Source: CAD feature listing. Evaluate the final solid. Frame: model axes, mm. Face numbers are marked on the shaded views. Coordinates: 2 decimals unless noted, no trailing zeros. Loops run counter-clockwise (first coordinate to the right, second up) from the corner with the lowest first, then second, coordinate; pieces in that order, holes last. Notation, with made-up numbers: (42, 43) - (59, 43) arc R18 ccw to (59, 59) - close; hole circle Ø5 at (60.5, -15). An arc over 180 degrees is marked (long way). Write item = value, one per line. Start each with the question number.
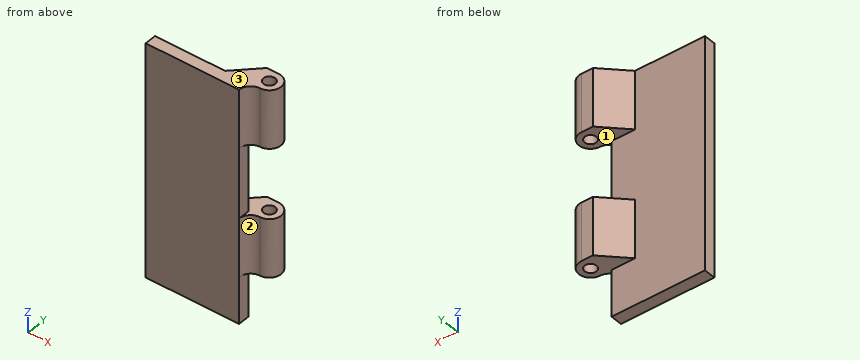
from build123d import *

# Parameters (mm, degrees)
SKETCH1_W              = 8
SKETCH1_H              = 20
BOSS_EXTRUDE1_DEPTH    = 1
SKETCH2_R              = 0.5
BOSS_EXTRUDE2_DEPTH    = 5
FILLET1_R              = 1
LPATTERN1_COUNT        = 2
LPATTERN1_PITCH        = 11
FILLET1_OF_LPATTERN1_R = 1


with BuildPart() as part:
    # Sketch1 → Boss-Extrude1 (new body)
    with BuildSketch(Plane(origin=(0, 0, 0), x_dir=(1, 0, 0), z_dir=(0, 1, 0))):
        with Locations((4, 10)):
            Rectangle(SKETCH1_W, SKETCH1_H)
    extrude(amount=BOSS_EXTRUDE1_DEPTH)

    # Sketch2 → Boss-Extrude2 (add)
    with BuildSketch(Plane.XY):
        with BuildLine():
            Line((8, 1), (9, 1))
            ThreePointArc((9, 1), (10, 2), (9, 3))
            Line((9, 3), (8, 3))
            Line((8, 3), (6, 1))
            Line((6, 1), (8, 1))
        make_face()
        with Locations((9, 2)):
            Circle(SKETCH2_R, mode=Mode.SUBTRACT)
    boss_extrude2 = extrude(amount=-BOSS_EXTRUDE2_DEPTH)

    # Fillet1
    fillet1_edges = [part.edges().sort_by_distance(p)[0] for p in [
        (8, 1, -2.5),
    ]]
    fillet(fillet1_edges, radius=FILLET1_R - 0.0001)  # a hair under: the kernel refuses the full size

    # LPattern1: Boss-Extrude2 ×2
    with Locations(*[(0, 0, -i * LPATTERN1_PITCH) for i in range(1, LPATTERN1_COUNT)]):
        add(boss_extrude2)

    # Fillet1 of LPattern1
    fillet1_of_lpattern1_edges = [part.edges().sort_by_distance(p)[0] for p in [
        (8, 1, -13.5),
    ]]
    fillet(fillet1_of_lpattern1_edges, radius=FILLET1_OF_LPATTERN1_R - 0.0001)  # a hair under: the kernel refuses the full size


solid = part.part
Item 1: Cut plane B-B (x = 5). Return the cut outline in (y, z).
Item 2: Material intervals for L1, parallel to Y at x = 9, z = -1.55; L2, parallel to Z at x = 7.5, y = 2.45; L3, parallel to Y at x = 1.75, z = -4.75, sorted ascending. Write a range as [from, to].
Item 3: Cut plane A-A (y = 2). Return the cut outline in (x, z), then the cut area to 3 significant figures.
Item 4: Draft query along Z for the marked faces 1, 2 and 3. Return one class per face: released by +Z, released by -Z, zero draft, split by the parting line, or undercut.
Item 5: First-contact query: pin 1 (3 mm diameter, centred on x = 5.5, z = -12, fed in from +Y); pin 2 (5 mm diameter, centred on x = 3, z = -7.5, fed in from +Y); pin 3 (0.9 mm diameter, centred on x = 8, y = 2, fed in from -Z). Flat tips, straight axial feed; report the tip coordinate or a pass-through.
Item 6: Cut plane D-D (z = -9.25). Return the cut outline in (x, y).
Item 7: Cut plane C-C (y = 0.7). Return the cut outline in (x, z), then the cut area to 3 significant figures.
Responses:
q1.outline = (0, -20) - (1, -20) - (1, 0) - (0, 0) - close
q2.L1 = [1, 1.5], [2.5, 3]
q2.L2 = [-16, -11], [-5, 0]
q2.L3 = [0, 1]
q3.outline = (7, -16) - (8.5, -16) - (8.5, -11) - (7, -11) - close; (7, -5) - (8.5, -5) - (8.5, 0) - (7, 0) - close; (9.5, -16) - (10, -16) - (10, -11) - (9.5, -11) - close; (9.5, -5) - (10, -5) - (10, 0) - (9.5, 0) - close
q3.area = 20.0 mm2
q4.face_1 = undercut
q4.face_2 = zero draft
q4.face_3 = released by +Z
q5.pin_1 = 2
q5.pin_2 = 1
q5.pin_3 = -16
q6.outline = (0, 0) - (8, 0) - (8, 1) - (0, 1) - close
q7.outline = (0, -20) - (8, -20) - (8, -16) - (8.29, -16) - (8.29, -11) - (8, -11) - (8, -5) - (8.29, -5) - (8.29, 0) - (0, 0) - close
q7.area = 163 mm2
